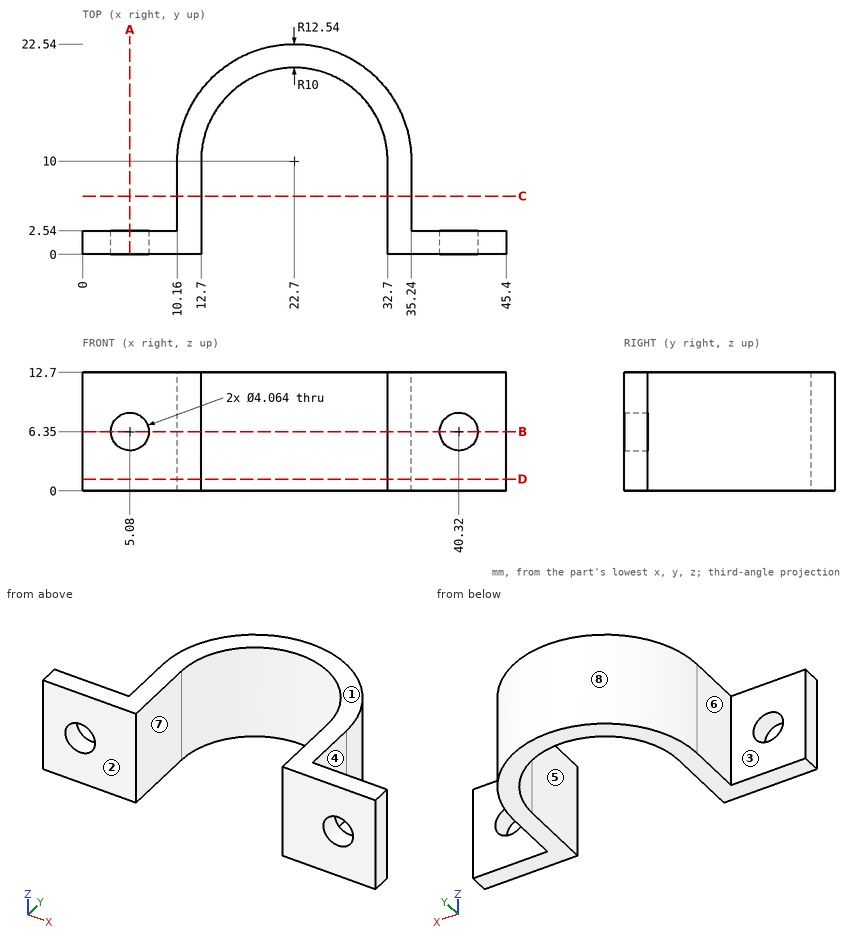
Geometry check sheet. Reference: drawing and pictorial views, mm from the part's lowest x, y, z. A direction names the side the tool comes from. Round coordinates to 2 decimals unless told otherwise and drop trailing zeros. Write each loop counter-clockwise with the first axis right and the second up, starting at its lowest first coordinate (ties: lowest second). Pieces come first, ordered by that corner, then holes.
(1) Material ranges on line 1 (X direction, y = 1.2, z = 6.35); line 2 (X direction, y = 2.25, z = 10.5); line 3 (Z direction, x = 40.5, y = 1.75), recorded low to high.
Returned:
line 1: x = 0 to 3.05, 7.11 to 12.7, 32.7 to 38.29, 42.35 to 45.4
line 2: x = 0 to 12.7, 32.7 to 45.4
line 3: z = 0 to 4.33, 8.37 to 12.7
(2) Depth check by flat-ended pin: pin 1 Ø5 at (x, z) = (39, 5) entering from +Y; pin 2 Ø4 at (x, z) = (19.5, 3) entering from -Y; pin 3 Ø6 at (y, z) = (7, 6.5) entering from -X. Enter the tip coordinate at first touch or a pass-through.
Returned:
pin 1: stops at y = 2.54
pin 2: stops at y = 18.54
pin 3: stops at x = 10.16
(3) Section check A-A (x = 5.08). Enter the section's corners in (y, z), plus the area to 3 significant figures.
Returned:
outline: (0, 0) - (2.54, 0) - (2.54, 4.32) - (0, 4.32) - close; (0, 8.38) - (2.54, 8.38) - (2.54, 12.7) - (0, 12.7) - close
area: 21.9 mm2
(4) Section check B-B (z = 6.35). Enter the section's corners in (x, y), plus the area to 3 significant figures.
Returned:
outline: (0, 0) - (3.05, 0) - (3.05, 2.54) - (0, 2.54) - close; (7.11, 0) - (12.7, 0) - (12.7, 10) arc R10 cw to (32.7, 10) - (32.7, 0) - (38.29, 0) - (38.29, 2.54) - (35.24, 2.54) - (35.24, 10) arc R12.54 ccw to (10.16, 10) - (10.16, 2.54) - (7.11, 2.54) - close; (42.35, 0) - (45.4, 0) - (45.4, 2.54) - (42.35, 2.54) - close
area: 172 mm2
(5) Access from +Z, -Z, +X, -X, +Y, -Y to the whole of each face (thin tool, end or side, straight path). Record for the marked faces 1, 2, 3, 4 and 5.
Returned:
face 1: +Z, +X, -X, +Y, -Y
face 2: +Z, -Z, +X, -X, -Y
face 3: +Z, -Z, -X, +Y
face 4: +Z, -Z, +X, +Y
face 5: +Z, -Z, -Y
(6) Section check C-C (y = 6.25). Enter the section's corners in (x, z), plus the area to 3 significant figures.
Returned:
outline: (10.16, 0) - (12.7, 0) - (12.7, 12.7) - (10.16, 12.7) - close; (32.7, 0) - (35.24, 0) - (35.24, 12.7) - (32.7, 12.7) - close
area: 64.5 mm2
(7) Section check D-D (z = 1.25). Enter the section's corners in (x, y).
Returned:
outline: (0, 0) - (12.7, 0) - (12.7, 10) arc R10 cw to (32.7, 10) - (32.7, 0) - (45.4, 0) - (45.4, 2.54) - (35.24, 2.54) - (35.24, 10) arc R12.54 ccw to (10.16, 10) - (10.16, 2.54) - (0, 2.54) - close
(8) Mould release check, pull along X, two halves, no side actions. Record for the marked faces 6, 7 and 8: pulls with the +X half, pulls with the -X half, needs draft (parallel to the pull), parting line crosses it, or undercut.
Returned:
face 6: pulls with the -X half
face 7: undercut
face 8: parting line crosses it
